Read the model definition and answer for the solid it produces. Units are mm, in the model's axes. Face numbers are marked on the shaded views. A direction names the side the tool comes from. Give positions to 0.01 mm unless a question says otherwise; leave off trailing zeros. Answer as CSV lines item,"result". Start each with the question number.
```python
from build123d import *

# Parameters (mm, degrees)
CREATION_EXTRUDE_DEPTH = 130.901699304
CREATION_EXTRUDE_TAPER = -26.56505118
SKETCH2_OUTSIDE_W      = 455.432
SKETCH2_OUTSIDE_H      = 443.246
CREATION_CUT_DEPTH     = 130.901699304
CREATION_CUT_TAPER     = 26.56505118
CUT_EXTRUDE_B_DEPTH    = 50.8
C_INV_DEPTH            = 50.8
CUT_EXTRUDE_D_DEPTH    = 50.8
D_INV_DEPTH            = 50.8
CUT_EXTRUDE_E_DEPTH    = 50.8
E_INV_DEPTH            = 50.8
CUT_EXTRUDE_F_DEPTH    = 50.8
F_INV_DEPTH            = 50.8
SKETCH17_R             = 6.35
BOSS_EXTRUDE1_DEPTH    = 127


with BuildPart() as part:
    # Sketch1 → creation_extrude (new body)
    with BuildSketch(Plane(origin=(0, 0, 0), x_dir=(1, 0, 0), z_dir=(0, 1, 0))):
        Polygon((0, 49.999999949), (-47.552825766, 15.450849703), (-29.389262585, -40.450849677), (29.389262585, -40.450849677), (47.552825766, 15.450849703), align=None)
    extrude(amount=CREATION_EXTRUDE_DEPTH, taper=CREATION_EXTRUDE_TAPER)

    # Sketch2 outside → creation_cut (cut)
    with BuildSketch(Plane(origin=(0, 130.901699304, 0), x_dir=(1, 0, 0), z_dir=(0, 1, 0))):
        with Locations((0, 12.5)):
            Rectangle(SKETCH2_OUTSIDE_W, SKETCH2_OUTSIDE_H)
        Polygon((0, -49.999999949), (47.552825766, -15.450849703), (29.389262585, 40.450849677), (-29.389262585, 40.450849677), (-47.552825766, -15.450849703), align=None, mode=Mode.SUBTRACT)
    extrude(amount=-CREATION_CUT_DEPTH, taper=CREATION_CUT_TAPER, mode=Mode.SUBTRACT)

    # Sketch5 → Cut-Extrude B (cut)
    with BuildSketch(Plane(origin=(0, 42.360679738, -84.721359466), x_dir=(-1, 0, 0), z_dir=(-9.08060963965006e-15, 0.4472135955455734, -0.8944271909771081))):
        Polygon((-42.797543189, 44.635254864), (1e-09, 13.541019643), (42.79754319, 44.635254866), (26.450336325, 94.946784308), (-26.450336327, 94.946784307), align=None)
    extrude(amount=-CUT_EXTRUDE_B_DEPTH, mode=Mode.SUBTRACT)

    # Sketch8 → C_inv (cut)
    with BuildSketch(Plane(origin=(-30.776835339, -16.180339872, 9.999999989), x_dir=(0.2446443083020028, 0.12861712429362696, 0.9610446387935747), z_dir=(-0.8506508083303469, -0.4472135955455736, 0.27639320224297786))):
        Polygon((-31.935023341, 77.848060657), (-22.992425992, 25.708717357), (29.358450763, 18.101689683), (52.77047459, 65.539631327), (14.889024305, 102.464919293), align=None)
    extrude(amount=-C_INV_DEPTH, mode=Mode.SUBTRACT)

    # Sketch9 → Cut-Extrude D (cut)
    with BuildSketch(Plane(origin=(49.797965648, 42.360679738, 68.541019594), x_dir=(0.8506508083603209, -0.27639320226847824, -0.44721359547279954), z_dir=(0.5257311121057348, 0.44721359554557366, 0.7236067977315217))):
        Polygon((-4.184405192, 98.473361345), (-54.495934634, 82.126154482), (-54.495934634, 29.22548183), (-4.184405192, 12.878274966), (26.90983003, 55.675818156), align=None)
    extrude(amount=-CUT_EXTRUDE_D_DEPTH, mode=Mode.SUBTRACT)

    # Sketch10 → D_inv (cut)
    with BuildSketch(Plane(origin=(-19.021130306, -16.180339872, -26.180339859), x_dir=(-0.8506508083603233, 0.27639320226847536, 0.44721359547279665), z_dir=(-0.5257311121057309, -0.44721359554557344, -0.7236067977315247))):
        Polygon((31.995934659, 98.473361351), (-18.315594783, 82.126154488), (-18.315594783, 29.225481836), (31.995934659, 12.878274972), (63.090169881, 55.675818162), align=None)
    extrude(amount=-D_INV_DEPTH, mode=Mode.SUBTRACT)

    # Sketch11 → Cut-Extrude E (cut)
    with BuildSketch(Plane(origin=(-49.797965648, 42.360679738, 68.541019594), x_dir=(0.8506508083603298, 0.2763932022684677, 0.447213595472789), z_dir=(-0.5257311121057203, 0.44721359554557355, 0.7236067977315324))):
        Polygon((4.184405192, 98.473361345), (-26.90983003, 55.675818156), (4.184405192, 12.878274966), (54.495934634, 29.22548183), (54.495934634, 82.126154482), align=None)
    extrude(amount=-CUT_EXTRUDE_E_DEPTH, mode=Mode.SUBTRACT)

    # Sketch12 → E_inv (cut)
    with BuildSketch(Plane(origin=(19.021130306, -16.180339872, -26.180339859), x_dir=(-0.8506508083603274, -0.27639320226847064, -0.44721359547279194), z_dir=(0.5257311121057243, -0.44721359554557355, -0.7236067977315294))):
        Polygon((-31.99593466, 98.473361351), (-63.090169881, 55.67581816), (-31.995934658, 12.878274972), (18.315594784, 29.225481837), (18.315594782, 82.126154489), align=None)
    extrude(amount=-E_INV_DEPTH, mode=Mode.SUBTRACT)

    # Sketch13 → Cut-Extrude F (cut)
    with BuildSketch(Plane(origin=(-80.574800989, 42.360679738, -26.180339862), x_dir=(-0.24464430830199108, 0.12861712429362016, 0.9610446387935785), z_dir=(-0.8506508083303513, 0.4472135955455735, -0.2763932022429644))):
        Polygon((-12.522250637, 97.763517637), (-35.934274461, 50.325575991), (1.947175826, 13.400288027), (48.771223471, 38.017146666), (39.828626119, 90.156489966), align=None)
    extrude(amount=-CUT_EXTRUDE_F_DEPTH, mode=Mode.SUBTRACT)

    # Sketch14 → F_inv (cut)
    with BuildSketch(Plane(origin=(30.776835339, -16.180339872, 9.999999989), x_dir=(0.2446443083019939, -0.12861712429362177, -0.9610446387935776), z_dir=(0.8506508083303502, -0.4472135955455736, 0.2763932022429676))):
        Polygon((-29.358450768, 18.101689686), (22.992425988, 25.708717353), (31.935023344, 77.848060652), (-14.889024299, 102.464919294), (-52.770474589, 65.539631333), align=None)
    extrude(amount=-F_INV_DEPTH, mode=Mode.SUBTRACT)


with BuildPart() as body_2:
    # of the pieces the cut leaves, the one that is kept (f_inv_keep)
    add(part.part.solids().sort_by_distance((0, 0, -49.999999949))[0])

    # Sketch17 → Boss-Extrude1 (add)
    with BuildSketch(Plane(origin=(0, 130.901699304, 0), x_dir=(1, 0, 0), z_dir=(0, 1, 0))):
        with Locations(Location((0, 0, 0), (0, 0, 270))):
            Circle(SKETCH17_R)
    extrude(amount=-BOSS_EXTRUDE1_DEPTH)


solid = body_2.part
```
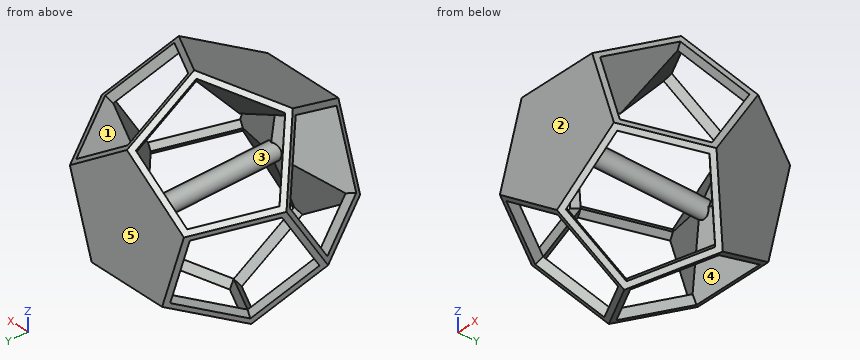
(1) A tool of negligible diameter and unlimited length cuts with its end or side. For the marked faces 3, 4 and 5, from which of +Z, -Z, +X, -X, +Y, -Y can it reach the whole face along a straight path? Write none if from no direction.
(2) The mould has two halves that part along X. Classify the marked faces 1 and 2: pulls with the +X half, pulls with the -X half, needs draft (parallel to the pull), parting line crosses it, or undercut.
(3) Find section A-A on y = 91.5. Give the number of separate pieces and of enclosed holes in the cut face, then the cut area to 3 significant figures.
(4) Find the intervals of material crossed by line 1 along Z through (x, y) = (1.5, 37); line 2 along Y through (x, z) = (1.5, -40); line 3 along Y through (x, z) = (-28.5, 22), in increasing order. Write a range as from..to.
(5) Each of these flat-tipped pins is pushed along its axis until it touches: P1, Ø1, axis at y = 38, z = 36, coming from the -X side; P2, Ø5, axis at y = 38, z = -24.5, coming from the +X side; P3, Ø3, axis at y = 79.5, z = -22.5, coming from the -X side. Where does it stop, or does it pass through?
Answer block:
1,face 3,"none"
1,face 4,"-Z"
1,face 5,"+Z, -Z, +X, -X, +Y"
2,face 1,"undercut"
2,face 2,"needs draft"
3,separate pieces,"5"
3,enclosed holes,"0"
3,area,"1,580 mm2"
4,line 1,"z = -71.78..-66.68, -6.17..6.17, 33.86..58.95"
4,line 2,"y = 0..8.13, 126.15..130.9"
4,line 3,"y = 0..7.8, 123.43..130.9"
5,P1,"stops at x = -6.25"
5,P2,"stops at x = 71.11"
5,P3,"stops at x = 38.27"
